Work out the finished part from the listing and answer in its coordinate system (mm). Face numbers are marked on the shaded views. A direction names the side the tool comes from. Give positions to 0.01 mm unless a question says otherwise; leave off trailing zeros. Loops run counter-clockwise (first coordinate to the right, second up) from the corner with the lowest first, then second, coordinate; pieces in that order, holes last.
```python
from build123d import *

# Parameters (mm, degrees)
SKETCH2_R           = 18.75
SKETCH2_R_2         = 1.6
BOSS_EXTRUDE1_DEPTH = 10
SKETCH3_R           = 9
BOSS_EXTRUDE2_DEPTH = 3
BOSS_EXTRUDE4_START = 3
SKETCH6_R           = 9
BOSS_EXTRUDE4_DEPTH = 3
SKETCH7_R           = 1.6
BOSS_EXTRUDE5_DEPTH = 1
FILLET2_R           = 0.05
SKETCH9_R           = 1.4
CUT_EXTRUDE1_DEPTH  = 10


with BuildPart() as part:
    # Sketch2 → Boss-Extrude1 (new body)
    with BuildSketch(Plane.XY):
        Circle(SKETCH2_R)
        with Locations((0, 14.5)):
            Circle(SKETCH2_R_2, mode=Mode.SUBTRACT)
        with Locations((12.557368355, 7.25)):
            Circle(SKETCH2_R_2, mode=Mode.SUBTRACT)
        with Locations((12.557368355, -7.25)):
            Circle(SKETCH2_R_2, mode=Mode.SUBTRACT)
        with Locations((0, -14.5)):
            Circle(SKETCH2_R_2, mode=Mode.SUBTRACT)
        with Locations((-12.557368355, -7.25)):
            Circle(SKETCH2_R_2, mode=Mode.SUBTRACT)
        with Locations((-12.557368355, 7.25)):
            Circle(SKETCH2_R_2, mode=Mode.SUBTRACT)
    extrude(amount=BOSS_EXTRUDE1_DEPTH)

    # Sketch3 → Boss-Extrude2 (add)
    with BuildSketch(Plane.XY.offset(10)):
        Circle(SKETCH3_R)
    extrude(amount=BOSS_EXTRUDE2_DEPTH)

    # Sketch6 → Boss-Extrude4 (add)
    with BuildSketch(Plane(origin=(0, 0, 0), x_dir=(-1, 0, 0), z_dir=(0, 0, -1)).offset(BOSS_EXTRUDE4_START)):
        with Locations(Location((0, 0, 0), (0, 0, 180))):
            Circle(SKETCH6_R)
    extrude(amount=-BOSS_EXTRUDE4_DEPTH)

    # Sketch7 → Boss-Extrude5 (add)
    with BuildSketch(Plane(origin=(0, 0, -3), x_dir=(-1, 0, 0), z_dir=(0, 0, -1))):
        Circle(SKETCH7_R)
    extrude(amount=BOSS_EXTRUDE5_DEPTH)

    # Fillet2
    fillet2_edges = [part.edges().sort_by_distance(p)[0] for p in [
        (1.6, 0, -4),
    ]]
    fillet(fillet2_edges, radius=FILLET2_R)

    # Sketch9 → Cut-Extrude1 (cut)
    with BuildSketch(Plane(origin=(0, 0, -4), x_dir=(-1, 0, 0), z_dir=(0, 0, -1))):
        Circle(SKETCH9_R)
    extrude(amount=-CUT_EXTRUDE1_DEPTH, mode=Mode.SUBTRACT)


solid = part.part
```
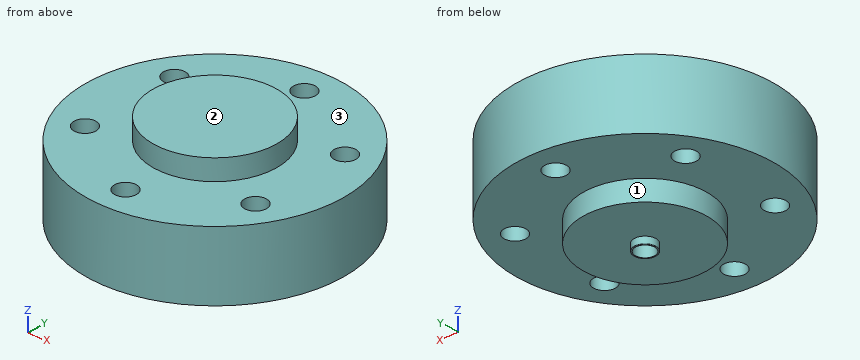
Q1. Which of the six approach directions +Z, -Z, +X, -X, +Y, -Y give full straight-line access (tool end or side, diameter ignored) to the marked faces 1, 2 and 3?
Q2. Section B-B on z = 1.75 is taken. Give the vertices of the cut face in (x, y), plus the area to 3 significant figures.
Q3. Given pin 1 (3 mm diameter, centred on y = -7.5, z = 10, fed in from -X); pin 2 (8 mm diameter, centred on y = 11, z = 9, fed in from +X); pin 3 (5 mm diameter, centred on x = 12.56, y = -7.25, fed in from -Z), each flat-ended and moving along its own axis, determine where each tip first touches the part or whether it passes through.
Q4. Section D-D on y = 7.25 is taken. Give the vertices of the cut face in (x, z), plus the area to 3 significant figures.
Q5. Consider line 1 along Y through (x, z) = (-1, 4.75); line 2 along Y through (x, z) = (0, 5.5); line 3 along Y through (x, z) = (12.5, 6). Determine where each line is inside the solid, lowest interval first.
Q6. Section A-A on y = -15 is taken. Give the vertices of the cut face in (x, z).
Q7. Section C-C on x = 8 is taken. Give the vertices of the cut face in (y, z), plus the area to 3 significant figures.
Check result:
1. face 1: -Z
1. face 2: +Z, +X, -X, +Y, -Y
1. face 3: +Z
2. outline: circle Ø37.5 at (0, 0); hole circle Ø3.2 at (-12.56, -7.25); hole circle Ø3.2 at (-12.56, 7.25); hole circle Ø3.2 at (0, -14.5); hole circle Ø3.2 at (0, 14.5); hole circle Ø2.8 at (0, 0); hole circle Ø3.2 at (12.56, -7.25); hole circle Ø3.2 at (12.56, 7.25)
2. area: 1,050 mm2
3. pin 1: stops at x = -17.76
3. pin 2: stops at x = 17.39
3. pin 3: stops at z = 0
4. outline: (-17.29, 0) - (-14.16, 0) - (-14.16, 10) - (-17.29, 10) - close; (-10.96, 0) - (-5.33, 0) - (-5.33, -3) - (5.33, -3) - (5.33, 0) - (10.96, 0) - (10.96, 10) - (5.33, 10) - (5.33, 13) - (-5.33, 13) - (-5.33, 10) - (-10.96, 10) - close; (14.16, 0) - (17.29, 0) - (17.29, 10) - (14.16, 10) - close
4. area: 346 mm2
5. line 1: y = -18.72 to -15.75, -13.25 to -0.98, 0.98 to 13.25, 15.75 to 18.72
5. line 2: y = -18.75 to -16.1, -12.9 to -1.4, 1.4 to 12.9, 16.1 to 18.75
5. line 3: y = -13.98 to -8.85, -5.65 to 5.65, 8.85 to 13.98
6. outline: (-11.25, 0) - (-1.52, 0) - (-1.52, 10) - (-11.25, 10) - close; (1.52, 0) - (11.25, 0) - (11.25, 10) - (1.52, 10) - close
7. outline: (-16.96, 0) - (-4.12, 0) - (-4.12, -3) - (4.12, -3) - (4.12, 0) - (16.96, 0) - (16.96, 10) - (4.12, 10) - (4.12, 13) - (-4.12, 13) - (-4.12, 10) - (-16.96, 10) - close
7. area: 389 mm2
